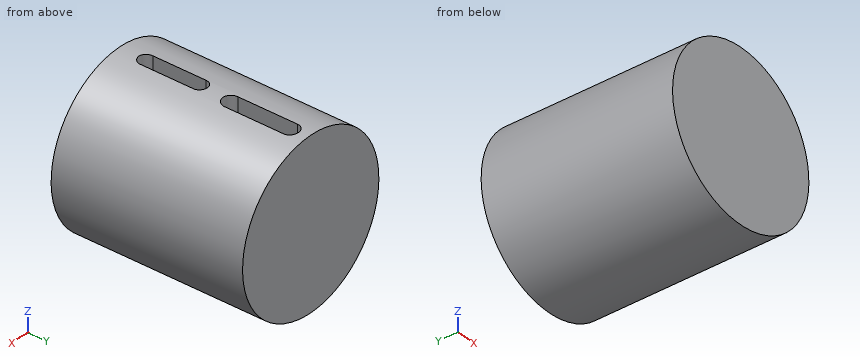
from build123d import *

# Parameters (mm, degrees)
SKETCH_3_R          = 27.991716744
EXTRUDE_1_DEPTH     = 65
CUT_EXTRUDE_1_DEPTH = 27
CUT_EXTRUDE_3_DEPTH = 50


with BuildPart() as part:
    # 草图3 → 凸台-拉伸1 (new body)
    with BuildSketch(Plane(origin=(0, 10, 0), x_dir=(1, 0, 0), z_dir=(0, 1, 0))):
        with Locations(Location((0, 0, 0), (0, 0, 270))):
            Circle(SKETCH_3_R)
    extrude(amount=EXTRUDE_1_DEPTH)

    # 草图4 → 切除-拉伸1 (cut)
    with BuildSketch(Plane.XY.offset(27.991716744)):
        with BuildLine():
            Line((3.744449093, 68.91896185), (3.744449093, 48.768976801))
            ThreePointArc((3.744449093, 48.768976801), (0.942846894, 45.967374602), (-1.858755305, 48.768976801))
            Line((-1.858755305, 48.768976801), (-1.858755305, 68.91896185))
            ThreePointArc((-1.858755305, 68.91896185), (0.942846894, 71.720564049), (3.744449093, 68.91896185))
        make_face()
    extrude(amount=-CUT_EXTRUDE_1_DEPTH, mode=Mode.SUBTRACT)

    # 草图6 → 切除-拉伸3 (cut)
    with BuildSketch(Plane.XY):
        with BuildLine():
            Line((2.586094338, 37.347060143), (2.586094338, 19.244399778))
            ThreePointArc((2.586094338, 19.244399778), (0, 16.658305441), (-2.586094338, 19.244399778))
            Line((-2.586094338, 19.244399778), (-2.586094338, 37.347060143))
            ThreePointArc((-2.586094338, 37.347060143), (0, 39.933154481), (2.586094338, 37.347060143))
        make_face()
    extrude(amount=CUT_EXTRUDE_3_DEPTH, mode=Mode.SUBTRACT)


solid = part.part
Source: CAD feature listing. Evaluate the final solid. Frame: model axes, mm. Give positions to 0.01 mm unless a question says otherwise; leave off trailing zeros. Order: outer loops, then holes, each group sorted by start corner. A loop starts at its lowest first (then second) coordinate and runs counter-clockwise, first axis right, second up. Notation, with made-up numbers: (69, 64) -> (94, 64) arc R17 cw to (94, 89) -> close; hole circle Ø3 at (-6, 26.25). An arc over 180 degrees is marked (long way). Write item = value, one per line.
Item 1: Section query B-B (x = 0). Output: boundary loops of the cut face in (y, z).
Check result:
outline = (10, -27.99) -> (75, -27.99) -> (75, 27.99) -> (71.56, 27.99) -> (71.56, 0.99) -> (46.13, 0.99) -> (46.13, 27.99) -> (39.93, 27.99) -> (39.93, 0) -> (16.66, 0) -> (16.66, 27.99) -> (10, 27.99) -> close
Item 2: Section query A-A (z = 21.5). Output: boundary loops of the cut face in (x, y).
Check result:
outline = (-17.92, 10) -> (17.92, 10) -> (17.92, 75) -> (-17.92, 75) -> close; hole (-2.59, 19.24) arc R2.59 ccw to (2.59, 19.24) -> (2.59, 37.35) arc R2.59 ccw to (-2.59, 37.35) -> close; hole (-1.86, 48.77) arc R2.8 ccw to (3.74, 48.77) -> (3.74, 68.92) arc R2.8 ccw to (-1.86, 68.92) -> close
Item 3: Ray query, probe 1 along Y at (x, z) = (3, 4); probe 2 along X at (y, z) = (69.5, 12); probe 3 along X at (y, z) = (49, 17). Return the intervals inside material, ascending.
Check result:
probe_1 = 10 to 46.87, 70.82 to 75
probe_2 = -25.29 to -1.8, 3.68 to 25.29
probe_3 = -22.24 to -1.86, 3.74 to 22.24
Item 4: Section query C-C (y = 55). Output: boundary loops of the cut face in (x, z), then the cut area to 3 significant figures.
Check result:
outline = (-1.86, 0.99) -> (-1.86, 27.93) arc R27.99 ccw (long way) to (3.74, 27.74) -> (3.74, 0.99) -> close
area = 2,310 mm²
Item 5: Contact query for flat-ended pins moving along their axis: pin 1 (9 mm diameter, centred on y = 31.5, z = 19, fed in from +X); pin 2 (8 mm diameter, centred on y = 18, z = -7, fed in from -X); pin 3 (16 mm diameter, centred on y = 57, z = 12.5, fed in from -X). Output: stop coordinate, or through.
Check result:
pin_1 = 23.94
pin_2 = -27.83
pin_3 = -27.63
Item 6: Section query D-D (z = -12.5). Output: boundary loops of the cut face in (x, y), then the cut area to 3 significant figures.
Check result:
outline = (-25.05, 10) -> (25.05, 10) -> (25.05, 75) -> (-25.05, 75) -> close
area = 3,260 mm²
